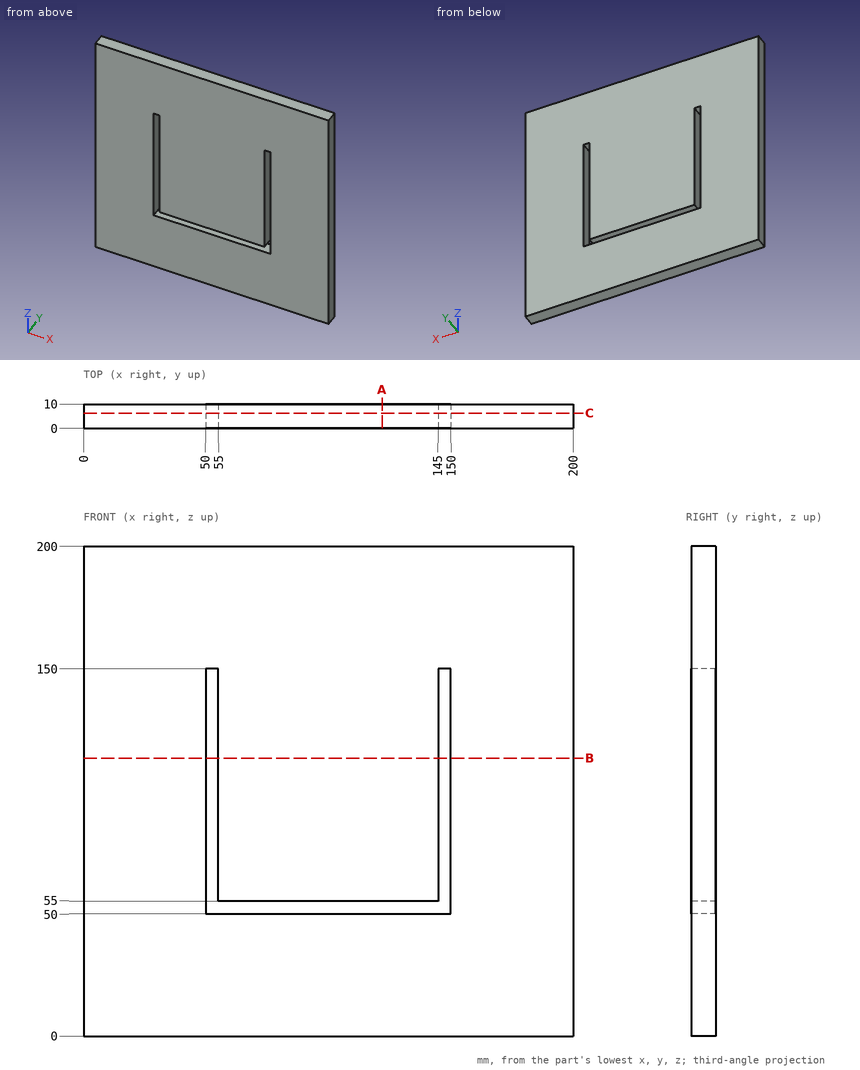
Input: dimensioned drawing with shaded views. Units: mm. Origin: part minimum x, y, z. Round coordinates to 2 decimals unless told otherwise and drop trailing zeros. Order: outer loops, then holes, each group sorted by start corner. A loop starts at its lowest first (then second) coordinate and runs counter-clockwise, first axis right, second up. Notation, with made-up numbers: (-23, 58) - (0, 58) arc R21 cw to (0, 79) - close; hole circle Ø1 at (88, 41.5). An arc over 180 degrees is marked (long way). Use CSV: the item, a comma, the result in double quotes. Start each with the question number.
Q1. Section query C-C (y = 6.25). Return loops of the section in (x, z), and give its area (4 significant figures).
Q2. Section query A-A (x = 122). Return loops of the section in (y, z).
Q3. Material intervals for line 1 along X through (y, z) = (9, 91); line 2 along Z through (x, y) = (107, 6); line 3 along Z through (x, y) = (52.5, 7.5), sorted ascending. Write a range as from..to.
Q4. Section query B-B (z = 113.5). Return loops of the section in (x, y).
Result set:
1,outline,"(0, 0) - (200, 0) - (200, 200) - (0, 200) - close; hole (50, 50) - (150, 50) - (150, 150) - (145, 150) - (145, 55) - (55, 55) - (55, 150) - (50, 150) - close"
1,area,"38,550 mm2"
2,outline,"(0, 0) - (10, 0) - (10, 50) - (0, 50) - close; (0, 55) - (10, 55) - (10, 200) - (0, 200) - close"
3,line 1,"x = 0..50, 55..145, 150..200"
3,line 2,"z = 0..50, 55..200"
3,line 3,"z = 0..50, 150..200"
4,outline,"(0, 0) - (50, 0) - (50, 10) - (0, 10) - close; (55, 0) - (145, 0) - (145, 10) - (55, 10) - close; (150, 0) - (200, 0) - (200, 10) - (150, 10) - close"
